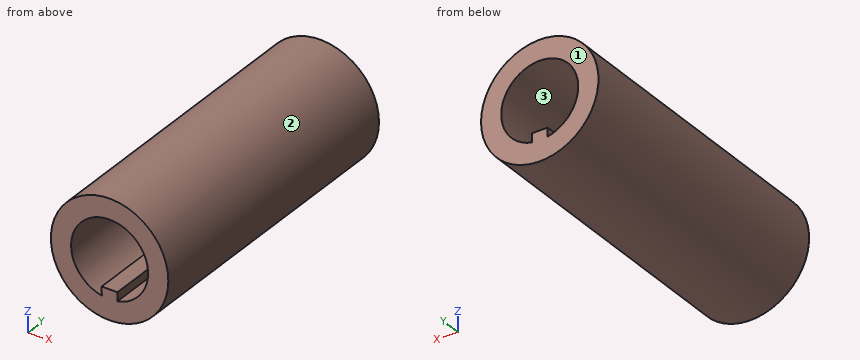
from build123d import *

# Parameters (mm, degrees)
F0_R     = 14.95
F1_DEPTH = 77


# Not quite as in the source:
# - a feature names something its author has since deleted; it is built from what else it names


with BuildPart() as f1:
    # F0 (on Front) → F1 (new body)
    with BuildSketch(Plane.XZ):
        Circle(F0_R)
        with BuildLine():
            ThreePointArc((-1.9898477157, -9.5958587978), (0, 9.8), (1.9898477157, -9.5958587978))
            Line((1.9898477157, -9.5958587978), (1.9898477157, -7.35))
            Line((1.9898477157, -7.35), (-2.0101522843, -7.35))
            Line((-2.0101522843, -7.35), (-1.9898477157, -9.5958587978))
        make_face(mode=Mode.SUBTRACT)
    extrude(amount=F1_DEPTH)


solid = f1.part
Source: CAD feature listing. Evaluate the final solid. Frame: model axes, mm. Face numbers are marked on the shaded views. Round coordinates to 2 decimals unless told otherwise and drop trailing zeros. Order: outer loops, then holes, each group sorted by start corner. A loop starts at its lowest first (then second) coordinate and runs counter-clockwise, first axis right, second up. Notation, with made-up numbers: (58.25, -23) - (109.25, -23) arc R30 cw to (109.25, 11) - close; hole circle Ø9 at (44.25, 18.5). An arc over 180 degrees is marked (long way). Use a Markdown table: item, result. Add a question column.
1. First-contact query: pin 1 (6 mm diameter, centred on x = 11, y = -62.5, fed in from -Z); pin 2 (2 mm diameter, centred on y = -64, z = 5, fed in from +X); pin 3 (1.1 mm diameter, centred on y = -47, z = -9, fed in from +X). Flat tips, straight axial feed; report the tip coordinate or a pass-through.
2. Section query B-B (x = 0). Return the cut outline in (y, z).
3. Section query C-C (y = -24.5). Return the cut outline in (x, z).
4. Mould query, pull axis Z, two halves, no side actions, for the marked faces 1, 2 and 3. Classes: +Z half, -Z half, draft (parallel to the pull), parting line (faces both ways), or undercut.
5. Line query: probe 1 along Z at (x, y) = (0, -37); probe 2 along Z at (x, y) = (-2.75, -27); probe 3 along X at (y, z) = (-73, 4.5). Output: solid intervals per line, ascending.
6. Section query D-D (z = -11.25). Return the cut outline in (x, y), then the cut area to 3 significant figures.
7. Section query A-A (z = 0). Return the cut outline in (x, y).
Derived:
| question | item | result |
|---|---|---|
| 1 | pin 1 | z = -12.63 |
| 1 | pin 2 | x = 14.4 |
| 1 | pin 3 | x = 12.33 |
| 2 | outline | (-77, -14.95) - (0, -14.95) - (0, -7.35) - (-77, -7.35) - close; (-77, 9.8) - (0, 9.8) - (0, 14.95) - (-77, 14.95) - close |
| 3 | outline | circle Ø29.9 at (0, 0); hole (-2.01, -7.35) - (1.99, -7.35) - (1.99, -9.6) arc R9.8 ccw (long way) to (-1.99, -9.6) - close |
| 4 | face 1 | draft |
| 4 | face 2 | parting line |
| 4 | face 3 | undercut |
| 5 | probe 1 | -14.95 to -7.35, 9.8 to 14.95 |
| 5 | probe 2 | -14.69 to -9.41, 9.41 to 14.69 |
| 5 | probe 3 | -14.26 to -8.71, 8.71 to 14.26 |
| 6 | outline | (-9.85, -77) - (9.85, -77) - (9.85, 0) - (-9.85, 0) - close |
| 6 | area | 1,520 mm2 |
| 7 | outline | (-14.95, -77) - (-9.8, -77) - (-9.8, 0) - (-14.95, 0) - close; (9.8, -77) - (14.95, -77) - (14.95, 0) - (9.8, 0) - close |
